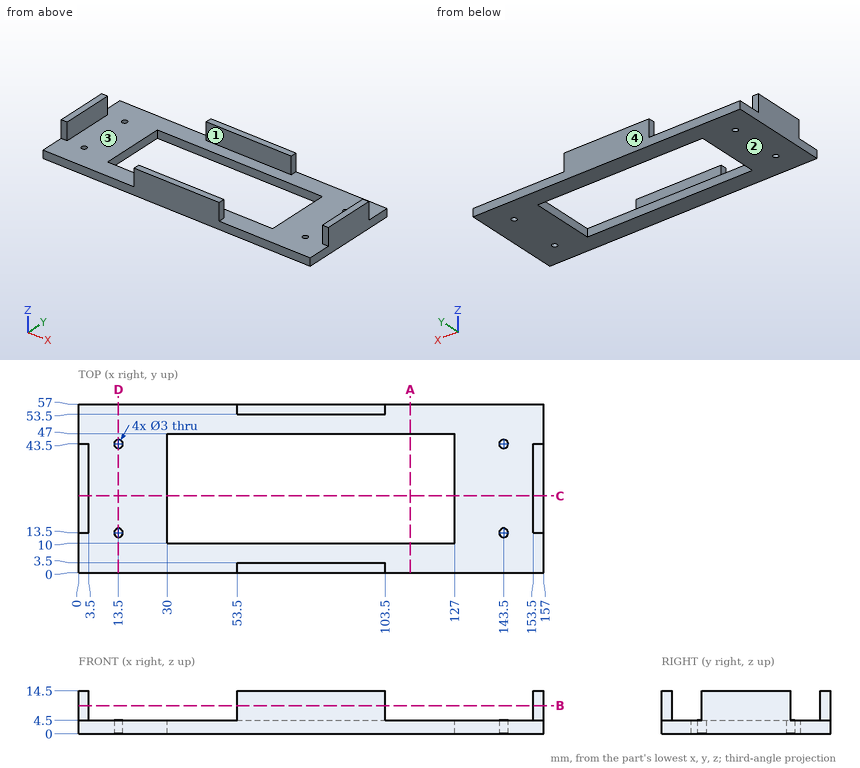
Geometry: see drawing. Coordinates: mm, zero at the bounding-box minimum. Give positions to 0.01 mm unless a question says otherwise; leave off trailing zeros. Write each loop counter-clockwise with the first axis right and the second up, starting at its lowest first coordinate (ties: lowest second). Pieces come first, ordered by that corner, then holes. Notation, with made-up numbers: M 56.25,53 L 104.25,53 A35 ccw 104.25,88 Z; hole C 24,7 d7. An arc over 180 degrees is marked long. Answer in a Markdown table with one row per item. Add a question column.
(1) First-contact query: pin 1 (1 mm diameter, centred on y = 1.5, z = 7.5, fed in from -X); pin 2 (1.8 mm diameter, centred on x = 2, z = 9.5, fed in from -Y); pin 3 (4 mm diameter, centred on y = 1, z = 9.5, fed in from +X). Flat tips, straight axial feed; report the tip coordinate or a pass-through.
(2) Section C-C on y = 26. Return loops of the section in (x, z), and give its area (3 significant figures).
(3) Section A-A on x = 112. Return loops of the section in (y, z).
(4) Mould query, pull axis Y, two halves, no side actions, for the marked faces 1, 2, 3 and 4. Classes: +Y half, -Y half, draft (parallel to the pull), parting line (faces both ways), or undercut.
(5) Section B-B on z = 9.5. Return loops of the section in (x, y), and give its area (3 significant figures).
(6) Section D-D on x = 13.5. Return loops of the section in (y, z).
(7) Ray query, line 1 (Y direction, x = 143.5, z = 2.8); line 2 (Y direction, x = 55, z = 9.75); line 3 (Y direction, x = 109.5, z = 1). Return the intervals inside material, ascending.
Result set:
| question | item | result |
|---|---|---|
| 1 | pin 1 | stops at x = 53.5 |
| 1 | pin 2 | stops at y = 13.5 |
| 1 | pin 3 | stops at x = 103.5 |
| 2 | outline | M 0,0 L 30,0 L 30,4.5 L 3.5,4.5 L 3.5,14.5 L 0,14.5 Z; M 127,0 L 157,0 L 157,14.5 L 153.5,14.5 L 153.5,4.5 L 127,4.5 Z |
| 2 | area | 340 mm^2 |
| 3 | outline | M 0,0 L 10,0 L 10,4.5 L 0,4.5 Z; M 47,0 L 57,0 L 57,4.5 L 47,4.5 Z |
| 4 | face 1 | undercut |
| 4 | face 2 | draft |
| 4 | face 3 | undercut |
| 4 | face 4 | +Y half |
| 5 | outline | M 0,13.5 L 3.5,13.5 L 3.5,43.5 L 0,43.5 Z; M 53.5,0 L 103.5,0 L 103.5,3.5 L 53.5,3.5 Z; M 53.5,53.5 L 103.5,53.5 L 103.5,57 L 53.5,57 Z; M 153.5,13.5 L 157,13.5 L 157,43.5 L 153.5,43.5 Z |
| 5 | area | 560 mm^2 |
| 6 | outline | M 0,0 L 12,0 L 12,4.5 L 0,4.5 Z; M 15,0 L 42,0 L 42,4.5 L 15,4.5 Z; M 45,0 L 57,0 L 57,4.5 L 45,4.5 Z |
| 7 | line 1 | y = 0 to 12, 15 to 42, 45 to 57 |
| 7 | line 2 | y = 0 to 3.5, 53.5 to 57 |
| 7 | line 3 | y = 0 to 10, 47 to 57 |
